Geometry check sheet. Reference: the model listing, model coordinates, mm. Round coordinates to 2 decimals unless told otherwise and drop trailing zeros. Write each loop counter-clockwise with the first axis right and the second up, starting at its lowest first coordinate (ties: lowest second). Pieces come first, ordered by that corner, then holes. Notation, with made-up numbers: M -21.5,38.5 L -2.5,38.5 A5 cw -2.5,42.5 Z; hole C -30.5,-11 d2. An arc over 180 degrees is marked long. Answer in a Markdown table with one row per item. Add a question column.
from build123d import *

# Parameters (mm, degrees)
F0_R     = 68.9281560168
F1_DEPTH = 54.864
F2_T     = -2.54
F4_R     = 0.9
F5_R     = 5.08


# Not quite as in the source:
# - a fillet or chamfer that OpenCascade refuses, or shapes differently, is made with other operations: its cross-section is extruded or revolved along the edge and cut away or added


with BuildPart() as f1:
    # F0 (on Top) → F1 (new body)
    with BuildSketch(Plane.XY):
        Circle(F0_R)
    extrude(amount=F1_DEPTH)

    # F2
    f2_openings = [f1.faces().sort_by_distance(p)[0] for p in [
        (0, 0, 54.864),
    ]]
    offset(amount=F2_T, openings=f2_openings)

    # F3: fillet of radius 5.08 on 1 edges, made by hand

    # F3_s1 → F3_t2 (revolve, cut)
    with BuildSketch(Plane.XZ):
        with BuildLine():
            ThreePointArc((68.9281560168, 50.4645909488), (68.247565068, 53.0045909488), (66.3881560168, 54.864))
            Line((66.3881560168, 54.864), (68.9281560168, 54.864))
            Line((68.9281560168, 54.864), (68.9281560168, 50.4645909488))
        make_face()
    revolve(axis=Axis((0, 0, 54.864), (0, 0, 1)), mode=Mode.SUBTRACT)

    # F4
    f4_edges = [f1.edges().sort_by_distance(p)[0] for p in [
        (-68.928156, 0, 0),
    ]]
    fillet(f4_edges, radius=F4_R)

    # F5
    f5_edges = [f1.edges().sort_by_distance(p)[0] for p in [
        (-66.388156, 0, 2.54),
    ]]
    fillet(f5_edges, radius=F5_R)


solid = f1.part
Item 1: Scan lines: probe 1 along Y at (x, z) = (0, 23); probe 2 along Z at (x, y) = (-30.5, 13.5); probe 3 along X at (y, z) = (17, 38.5). Record each from-to range of solid material in increasing order. Write a range as from..to.
Item 2: Gauge pin test, flat ends, axial feed: pin 1 Ø2 at (y, z) = (-26.5, 29) entering from +X; pin 2 Ø12 at (x, y) = (48, 9) entering from +Z; pin 3 Ø1.5 at (y, z) = (35, 49) entering from +X. Record the tip position at first contact, or that the pin passes through.
Item 3: Mould release check, pull along X, two halves, no side actions. Record for faces 1 (the cylindrical face through (-14.39, -64.81, 30.91)), 2 (the flat face through (-1, 1, 0)), 3 (the cylindrical face through (-54.7, -41.94, 25.34)), 4 (the flat face through (-1, 1, 2.54)): +X half, -X half, draft (parallel to the pull), parting line (faces both ways), or undercut.
Item 4: Section check A-A, the plane y = 0. Record the boundary of the cut face in (x, z), and give its area (3 significant figures).
Item 5: Section check B-B, the plane z = 12. Record the boundary of the cut face in (x, y), and give its area (3 significant figures).
Result sheet:
| question | item | result |
|---|---|---|
| 1 | probe 1 | y = -68.93..-66.39, 66.39..68.93 |
| 1 | probe 2 | z = 0..2.54 |
| 1 | probe 3 | x = -66.8..-64.17, 64.17..66.8 |
| 2 | pin 1 | stops at x = 64.04 |
| 2 | pin 2 | stops at z = 2.54 |
| 2 | pin 3 | stops at x = 59.82 |
| 3 | face 1 | undercut |
| 3 | face 2 | draft |
| 3 | face 3 | parting line |
| 3 | face 4 | undercut |
| 4 | outline | M -68.93,0.9 A0.9 ccw -68.03,0 L 68.03,0 A0.9 ccw 68.93,0.9 L 68.93,50.46 A5.08 ccw 66.39,54.86 L 66.39,7.62 A5.08 cw 61.31,2.54 L -61.31,2.54 A5.08 cw -66.39,7.62 L -66.39,54.86 A5.08 ccw -68.93,50.46 Z |
| 4 | area | 620 mm^2 |
| 5 | outline | C 0,0 d137.86; hole C 0,0 d132.78 |
| 5 | area | 1,080 mm^2 |
